Build history of the part. All positions in model axes, mm. Round coordinates to 2 decimals unless told otherwise and drop trailing zeros. Write each loop counter-clockwise with the first axis right and the second up, starting at its lowest first coordinate (ties: lowest second). Pieces come first, ordered by that corner, then holes. Notation, with made-up numbers: (-11.5, 52) -> (34.5, 52) arc R26 cw to (34.5, 79) -> close; hole circle Ø4 at (-19.5, 1). An arc over 180 degrees is marked (long way). Return JSON: item names as keys, results as strings.
from build123d import *

# Parameters (mm, degrees)
SKETCH1_W           = 20.32
SKETCH1_H           = 20.32
BOARD_OUTLINE_DEPTH = 1.6
SKETCH2_R           = 0.254
NPTH_DEPTH          = 29.78132728
SKETCH3_R           = 0.51
SKETCH3_R_2         = 0.45
PTH_DEPTH           = 29.78132728


with BuildPart() as part:
    # Sketch1 → Board_Outline (new body)
    with BuildSketch(Plane.XY):
        with Locations((10.16, 10.16)):
            Rectangle(SKETCH1_W, SKETCH1_H)
    extrude(amount=BOARD_OUTLINE_DEPTH)

    # Sketch2 → NPTH (cut, through all)
    with BuildSketch(Plane.XY):
        with Locations((9.525, 12.7)):
            Circle(SKETCH2_R)
        with Locations((11.43, 17.78)):
            Circle(SKETCH2_R)
        with Locations((10.16, 17.78)):
            Circle(SKETCH2_R)
        with Locations((10.795, 12.7)):
            Circle(SKETCH2_R)
        with Locations((3.175, 13.97)):
            Circle(SKETCH2_R)
        with Locations((8.89, 17.78)):
            Circle(SKETCH2_R)
        with Locations((15.7163, 10.16)):
            Circle(SKETCH2_R)
        with Locations((16.8275, 19.05)):
            Circle(SKETCH2_R)
        with Locations((8.255, 12.7)):
            Circle(SKETCH2_R)
        with Locations((17.9388, 10.16)):
            Circle(SKETCH2_R)
        with Locations((12.7, 12.7)):
            Circle(SKETCH2_R)
        with Locations((10.16, 1.27)):
            Circle(SKETCH2_R)
        with Locations((3.175, 16.51)):
            Circle(SKETCH2_R)
    extrude(amount=NPTH_DEPTH, mode=Mode.SUBTRACT)

    # Sketch3 → PTH (cut, through all)
    with BuildSketch(Plane.XY):
        with Locations((1.27, 1.27)):
            Circle(SKETCH3_R)
        with Locations((1.27, 3.81)):
            Circle(SKETCH3_R)
        with Locations((1.27, 6.35)):
            Circle(SKETCH3_R)
        with Locations((19.05, 16.51)):
            Circle(SKETCH3_R)
        with Locations((19.05, 13.97)):
            Circle(SKETCH3_R)
        with Locations((1.27, 16.51)):
            Circle(SKETCH3_R)
        with Locations((1.27, 13.97)):
            Circle(SKETCH3_R)
        with Locations((19.05, 1.27)):
            Circle(SKETCH3_R)
        with Locations((19.05, 3.81)):
            Circle(SKETCH3_R)
        with Locations((19.05, 6.35)):
            Circle(SKETCH3_R)
        with Locations((13.97, 8.89)):
            Circle(SKETCH3_R_2)
        with Locations((13.97, 1.27)):
            Circle(SKETCH3_R_2)
        with Locations((13.97, 11.43)):
            Circle(SKETCH3_R_2)
        with Locations((13.97, 19.05)):
            Circle(SKETCH3_R_2)
    extrude(amount=PTH_DEPTH, mode=Mode.SUBTRACT)


solid = part.part
Q1. Two-plate mould, pull along X, no slides. Class faces 1 (the flat face through (0, 10, 1)), 2 (the cylindrical face through (19.536, 14.123, 0.789)), 3 (the flat face through (20.32, 10, 1)): +X half, -X half, draft (parallel to the pull), parting line (faces both ways), or undercut.
Verdict:
{"face 1": "-X half", "face 2": "undercut", "face 3": "+X half"}
Q2. Saw through at D-D on z = 1. Count the separate pieces of the cut face and the enclosed holes in it, then the cut area to 3 significant figures.
Verdict:
{"separate pieces": "1", "enclosed holes": "27", "area": "400 mm²"}
Q3. Wall check: L1, parallel to X at y = 13.97, z = 1.15; L2, parallel to Y at x = 11.43, z = 1.05; L3, parallel to Y at x = 1.27, z = 0.6. Give the ranges that are in metal, low to high.
Verdict:
{"L1": "x = 0 to 0.76, 1.78 to 2.92, 3.43 to 18.54, 19.56 to 20.32", "L2": "y = 0 to 17.53, 18.03 to 20.32", "L3": "y = 0 to 0.76, 1.78 to 3.3, 4.32 to 5.84, 6.86 to 13.46, 14.48 to 16, 17.02 to 20.32"}
Q4. Saw through at A-A on y = 3.81. List the corners of the cut face in (x, z).
Verdict:
{"outline": "(0, 0) -> (0.76, 0) -> (0.76, 1.6) -> (0, 1.6) -> close; (1.78, 0) -> (18.54, 0) -> (18.54, 1.6) -> (1.78, 1.6) -> close; (19.56, 0) -> (20.32, 0) -> (20.32, 1.6) -> (19.56, 1.6) -> close"}
Q5. Saw through at C-C on x = 8.89. List the corners of the cut face in (y, z).
Verdict:
{"outline": "(0, 0) -> (17.53, 0) -> (17.53, 1.6) -> (0, 1.6) -> close; (18.03, 0) -> (20.32, 0) -> (20.32, 1.6) -> (18.03, 1.6) -> close"}
Q6. Saw through at B-B on y = 17.78. List the corners of the cut face in (x, z), then the cut area to 3 significant figures.
Verdict:
{"outline": "(0, 0) -> (8.64, 0) -> (8.64, 1.6) -> (0, 1.6) -> close; (9.14, 0) -> (9.91, 0) -> (9.91, 1.6) -> (9.14, 1.6) -> close; (10.41, 0) -> (11.18, 0) -> (11.18, 1.6) -> (10.41, 1.6) -> close; (11.68, 0) -> (20.32, 0) -> (20.32, 1.6) -> (11.68, 1.6) -> close", "area": "30.1 mm²"}
Q7. Pin check, flat tip, straight feed: pin 1 Ø0.9 at (x, y) = (1.27, 16.51) entering from -Z. Stop position of the tip, or through.
Verdict:
{"pin 1": "passes through"}
